```python
from build123d import *

# Parameters (mm, degrees)
BOSS_EXTRU_1_CORPS_DEPTH    = 263.5
CONG_1_R                    = 1.5
CONG_2_R                    = 0.4
CONG_4_R                    = 1
CONG_1_OF_SYM_TRIE_BRAS_R   = 1.5
CONG_2_OF_SYM_TRIE_BRAS_R   = 0.4
CONG_4_OF_SYM_TRIE_BRAS_R   = 1
SYM_TRIE_BRAS_DOUBLE_DEPTH  = 263.5
APR_S_TARODAGE_M6_R         = 3
ENL_V_MAT_FILETAGE_M6_DEPTH = 264.879233741


# Read off the part's stored shape, not the designer's step: Symétrie Bras double
with BuildPart() as part:
    # Esquisse4 → Boss.-Extru.1 Corps (new body)
    with BuildSketch(Plane(origin=(0, 0, 0), x_dir=(1, 0, 0), z_dir=(0, 1, 0))):
        Polygon((0, 0), (-4.5, 0), (-4.5, 3.625), (-6.875, 6), (-8.5, 6), (-8.5, 3), (-9.5, 3), (-9.5, 3.5), (-10, 3.5), (-10, 10), (-3.5, 10), (-3.5, 9.5), (-3, 9.5), (-3, 8.5), (-6, 8.5), (-6, 6.875), (-3.625, 4.5), (0, 4.5), align=None)
    boss_extru_1_corps = extrude(amount=BOSS_EXTRU_1_CORPS_DEPTH)

    # Congé1
    cong_1_edges = [part.edges().sort_by_distance(p)[0] for p in [
        (-10, 131.75, -10),
    ]]
    fillet(cong_1_edges, radius=CONG_1_R)

    # Congé2
    cong_2_edges = [part.edges().sort_by_distance(p)[0] for p in [
        (-8.5, 131.75, -6),
        (-6, 131.75, -8.5),
    ]]
    fillet(cong_2_edges, radius=CONG_2_R)

    # Congé4
    cong_4_edges = [part.edges().sort_by_distance(p)[0] for p in [
        (-4.5, 131.75, -3.625),
        (-6.875, 131.75, -6),
        (-6, 131.75, -6.875),
        (-3.625, 131.75, -4.5),
    ]]
    fillet(cong_4_edges, radius=CONG_4_R)

    # Symétrie Bras: Boss.-Extru.1 Corps across plane
    add(boss_extru_1_corps.mirror(Plane(origin=(0, 263.5, -4.5), x_dir=(0, 0, 1), z_dir=(-1, 0, 0))))

    # Congé1 of Symétrie Bras
    cong_1_of_sym_trie_bras_edges = [part.edges().sort_by_distance(p)[0] for p in [
        (10, 131.75, -10),
    ]]
    fillet(cong_1_of_sym_trie_bras_edges, radius=CONG_1_OF_SYM_TRIE_BRAS_R)

    # Congé2 of Symétrie Bras
    cong_2_of_sym_trie_bras_edges = [part.edges().sort_by_distance(p)[0] for p in [
        (8.5, 131.75, -6),
        (6, 131.75, -8.5),
    ]]
    fillet(cong_2_of_sym_trie_bras_edges, radius=CONG_2_OF_SYM_TRIE_BRAS_R)

    # Congé4 of Symétrie Bras
    cong_4_of_sym_trie_bras_edges = [part.edges().sort_by_distance(p)[0] for p in [
        (4.5, 131.75, -3.625),
        (6.875, 131.75, -6),
        (6, 131.75, -6.875),
        (3.625, 131.75, -4.5),
    ]]
    fillet(cong_4_of_sym_trie_bras_edges, radius=CONG_4_OF_SYM_TRIE_BRAS_R)

    # Symétrie Bras double outline → Symétrie Bras double (add)
    with BuildSketch(Plane(origin=(0, 0, 0), x_dir=(1, 0, 0), z_dir=(0, 1, 0))):
        with BuildLine():
            ThreePointArc((7.289213562, -6), (6.90653013, -5.923879533), (6.582106781, -5.707106781))
            Line((6.582106781, -5.707106781), (4.792893219, -3.917893219))
            ThreePointArc((4.792893219, -3.917893219), (4.576120467, -3.59346987), (4.5, -3.210786438))
            Line((4.5, -3.210786438), (4.5, 0))
            Line((4.5, 0), (-4.5, 0))
            Line((-4.5, 0), (-4.5, -3.210786438))
            ThreePointArc((-4.5, -3.210786438), (-4.576120467, -3.59346987), (-4.792893219, -3.917893219))
            Line((-4.792893219, -3.917893219), (-6.582106781, -5.707106781))
            ThreePointArc((-6.582106781, -5.707106781), (-6.90653013, -5.923879533), (-7.289213562, -6))
            Line((-7.289213562, -6), (-8.1, -6))
            ThreePointArc((-8.1, -6), (-8.382842712, -5.882842712), (-8.5, -5.6))
            Line((-8.5, -5.6), (-8.5, -3))
            Line((-8.5, -3), (-9.5, -3))
            Line((-9.5, -3), (-9.5, -3.5))
            Line((-9.5, -3.5), (-10, -3.5))
            Line((-10, -3.5), (-10, -8.5))
            ThreePointArc((-10, -8.5), (-9.560660172, -9.560660172), (-8.5, -10))
            Line((-8.5, -10), (-3.5, -10))
            Line((-3.5, -10), (-3.5, -9.5))
            Line((-3.5, -9.5), (-3, -9.5))
            Line((-3, -9.5), (-3, -8.5))
            Line((-3, -8.5), (-5.6, -8.5))
            ThreePointArc((-5.6, -8.5), (-5.882842712, -8.382842712), (-6, -8.1))
            Line((-6, -8.1), (-6, -7.289213562))
            ThreePointArc((-6, -7.289213562), (-5.923879533, -6.90653013), (-5.707106781, -6.582106781))
            Line((-5.707106781, -6.582106781), (-3.917893219, -4.792893219))
            ThreePointArc((-3.917893219, -4.792893219), (-3.59346987, -4.576120467), (-3.210786438, -4.5))
            Line((-3.210786438, -4.5), (3.210786438, -4.5))
            ThreePointArc((3.210786438, -4.5), (3.59346987, -4.576120467), (3.917893219, -4.792893219))
            Line((3.917893219, -4.792893219), (5.707106781, -6.582106781))
            ThreePointArc((5.707106781, -6.582106781), (5.923879533, -6.90653013), (6, -7.289213562))
            Line((6, -7.289213562), (6, -8.1))
            ThreePointArc((6, -8.1), (5.882842712, -8.382842712), (5.6, -8.5))
            Line((5.6, -8.5), (3, -8.5))
            Line((3, -8.5), (3, -9.5))
            Line((3, -9.5), (3.5, -9.5))
            Line((3.5, -9.5), (3.5, -10))
            Line((3.5, -10), (8.5, -10))
            ThreePointArc((8.5, -10), (9.560660172, -9.560660172), (10, -8.5))
            Line((10, -8.5), (10, -3.5))
            Line((10, -3.5), (9.5, -3.5))
            Line((9.5, -3.5), (9.5, -3))
            Line((9.5, -3), (8.5, -3))
            Line((8.5, -3), (8.5, -5.6))
            ThreePointArc((8.5, -5.6), (8.382842712, -5.882842712), (8.1, -6))
            Line((8.1, -6), (7.289213562, -6))
        make_face()
    extrude(amount=SYM_TRIE_BRAS_DOUBLE_DEPTH)

    # Après tarodage M6 → Enlèv. mat.-Filetage M6 (cut, through all)
    with BuildSketch(Plane.XZ):
        with Locations(Location((0, 0, 0), (0, 0, 270))):
            Circle(APR_S_TARODAGE_M6_R)
    extrude(amount=-ENL_V_MAT_FILETAGE_M6_DEPTH, mode=Mode.SUBTRACT)


solid = part.part
```
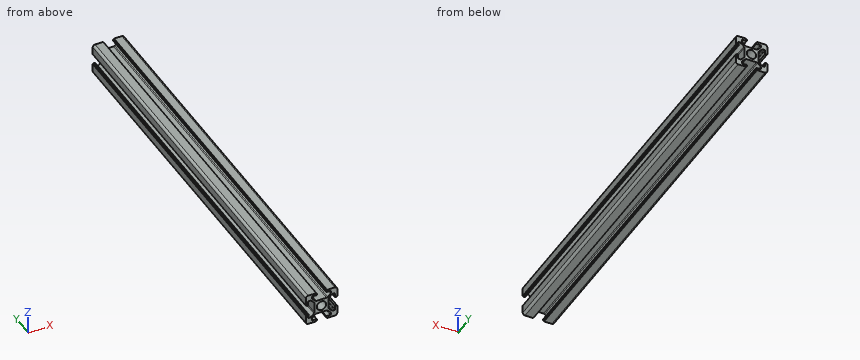
Verification items for the finished model (mm, model axes). Coordinates: 2 decimals unless noted, no trailing zeros. Order: outer loops, then holes, each group sorted by start corner. A loop starts at its lowest first (then second) coordinate and runs counter-clockwise, first axis right, second up. Notation, with made-up numbers: (-20, -40) -> (-10, -40) arc R8 ccw to (-10, -34) -> close; hole circle Ø3 at (-0.75, -19.75). An arc over 180 degrees is marked (long way). Put each result on its own line as item: value. Start each with the question number.
1) Cross-section at B-B (x = 0). Enter the section's corners in (y, z).
2) Material ranges on L1, parallel to X at y = 155.5, z = -7.5; L2, parallel to Z at x = 5.5, y = 77 (3 decimals); L3, parallel to X at y = 204.5, z = 0, recorded low to high.
3) Cross-section at A-A (z = 0). Enter the section's corners in (x, y), plus the area to 4 significant figures.
4) Go/stop test with flat-tipped pins: pin 1 (4 mm diameter, centred on x = 6, z = 5.5, fed in from -Y); pin 2 (1.5 mm diameter, centred on x = -4, z = -6.5, fed in from -Y); pin 3 (0.8 mm diameter, centred on x = 9, y = 101, fed in from +Z); pin 4 (0.6 mm diameter, centred on y = 181, z = -3, fed in from +X). Record where each tip stops, or that it passes through.
Geometry check:
1. outline: (0, -4.5) -> (263.5, -4.5) -> (263.5, -3) -> (0, -3) -> close; (0, 3) -> (263.5, 3) -> (263.5, 4.5) -> (0, 4.5) -> close
2. L1: x = -10 to -6, 6 to 10
2. L2: z = -10 to -8.5, -6.375 to -4.625, 4.625 to 6.375, 8.5 to 10
2. L3: x = -4.5 to -3, 3 to 4.5
3. outline: (-4.5, 0) -> (-3, 0) -> (-3, 263.5) -> (-4.5, 263.5) -> close; (3, 0) -> (4.5, 0) -> (4.5, 263.5) -> (3, 263.5) -> close
3. area: 790.5 mm^2
4. pin 1: stops at y = 0
4. pin 2: passes through
4. pin 3: stops at z = 10
4. pin 4: stops at x = 9.5
